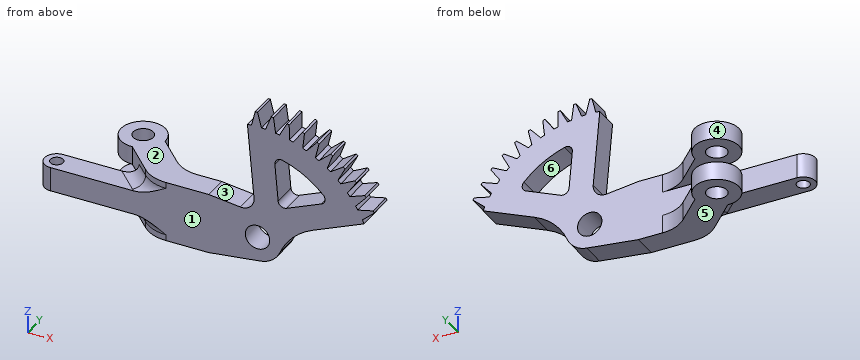
from build123d import *

# Parameters (mm, degrees)
SKETCH1_R           = 1.6500000000000001
BOSS_EXTRUDE1_DEPTH = 5
CUT_EXTRUDE1_DEPTH  = 22.617643257302586
SKETCH4_R           = 2.000000000000003
BOSS_EXTRUDE2_DEPTH = 4
SKETCH5_R           = 1.0500000000000005
BOSS_EXTRUDE3_DEPTH = 2
CUT_EXTRUDE2_REACH  = 52.658
CIRPATTERN1_COUNT   = 11
CIRPATTERN1_ANGLE   = 70.00000000000016
CUT_EXTRUDE3_DEPTH  = 4
FILLET1_R           = 6
FILLET2_R           = 2
CUT_EXTRUDE4_REACH  = 51.172


with BuildPart() as part:
    # Sketch1 → Boss-Extrude1 (new, symmetric)
    with BuildSketch(Plane.XY):
        with BuildLine():
            Line((6.464466094067297, -10), (16, -10))
            Line((16, -10), (16, -5.999999999999998))
            Line((16, -5.999999999999998), (9.535533905932775, -5.999999999999998))
            Line((9.535533905932775, -5.999999999999998), (3.6482589098755183, -0.11272500394276944))
            ThreePointArc((3.6482589098755183, -0.11272500394276944), (-2.580939751330903, 2.5809397513308943), (0.11272500394278592, -3.6482589098755174))
            Line((0.11272500394278592, -3.6482589098755174), (6.464466094067297, -10))
        make_face()
        Circle(SKETCH1_R, mode=Mode.SUBTRACT)
    extrude(amount=BOSS_EXTRUDE1_DEPTH, both=True)

    # Sketch3 → Cut-Extrude1 (cut, through all)
    with BuildSketch(Plane.XZ.offset(10)):
        Polygon((6.464466094067297, 2.000000000000001), (-3.6500000000000012, 1.9999999999999996), (-3.650000000000001, -2.0000000000000004), (6.464466094067298, -1.9999999999999991), align=None)
    extrude(amount=-CUT_EXTRUDE1_DEPTH, mode=Mode.SUBTRACT)

    # Sketch4 → Boss-Extrude2 (add)
    with BuildSketch(Plane.XZ.offset(10)):
        with BuildLine():
            Line((16, 5), (16, -5))
            Line((16, -5), (21.19546555409763, -4.369618467658506))
            Line((21.19546555409763, -4.369618467658506), (24.481798594453377, -3.970877751125406))
            ThreePointArc((24.481798594453377, -3.970877751125406), (26.41654324887739, -3.187525486377344), (27.693251449070946, -1.5361945625263))
            ThreePointArc((27.693251449070946, -1.5361945625263), (29.829731429750588, 1.668713133124987), (33.01906878685553, 3.8283675656823353))
            Line((33.01906878685553, 3.8283675656823353), (43.79085434922743, 8.400719262519475))
            ThreePointArc((43.79085434922743, 8.400719262519475), (35.07331861056618, 18.429096965095408), (22.126151530925494, 21.418186008972544))
            Line((22.126151530925494, 21.418186008972544), (23.428754247507808, 6.529368828716514))
            ThreePointArc((23.428754247507808, 6.529368828716514), (22.82671005925236, 4.917371632507108), (21.19546555409763, 4.369618467658506))
            Line((21.19546555409763, 4.369618467658506), (16, 5))
        make_face()
        with Locations(Location((24, 0, 0), (0, 0, 270))):
            Circle(SKETCH4_R, mode=Mode.SUBTRACT)
    extrude(amount=-BOSS_EXTRUDE2_DEPTH)

    # Sketch5 → Boss-Extrude3 (add, symmetric)
    with BuildSketch(Plane.XY):
        with BuildLine():
            Line((6.464466094067297, -10), (-10, -10.000000000000002))
            ThreePointArc((-10, -10.000000000000002), (-11.999999999999998, -8), (-9.999999999999998, -6.000000000000002))
            Line((-9.999999999999998, -6.000000000000002), (9.535533905932775, -5.999999999999998))
            Line((9.535533905932775, -5.999999999999998), (16, -5.999999999999998))
            Line((16, -5.999999999999998), (16, -10))
            Line((16, -10), (6.464466094067297, -10))
        make_face()
        with Locations((-9.999999999999998, -8.000000000000002)):
            Circle(SKETCH5_R, mode=Mode.SUBTRACT)
    extrude(amount=BOSS_EXTRUDE3_DEPTH, both=True)

    # Sketch6 → Cut-Extrude2 (cut, up to next)
    with BuildSketch(Plane.XZ.offset(10), mode=Mode.PRIVATE) as cut_extrude2_sk1:
        with BuildLine():
            Line((41.21984795369632, 8.029746973073365), (43.15664027004987, 9.760795744400328))
            ThreePointArc((43.15664027004987, 9.760795744400328), (43.324071995432064, 9.424979655965245), (43.48561742128794, 9.086292627425122))
            ThreePointArc((43.48561742128794, 9.086292627425122), (43.64122733931588, 8.744837826129787), (43.79085434922743, 8.40071926251947))
            ThreePointArc((43.79085434922743, 8.40071926251947), (43.93445287318589, 8.054041758442194), (44.071979169689804, 7.704910915224042))
            Line((44.071979169689804, 7.704910915224042), (41.48959221559633, 7.42389144129628))
            ThreePointArc((41.48959221559633, 7.42389144129628), (41.357363695209386, 7.72799621844028), (41.21984795369632, 8.029746973073365))
        make_face()
    cut_extrude2_tool1 = extrude(cut_extrude2_sk1.sketch, amount=-CUT_EXTRUDE2_REACH, mode=Mode.PRIVATE) & part.part
    cut_extrude2 = cut_extrude2_tool1.solids().sort_by_distance((42.701484, -10, 8.326437))[0]
    add(cut_extrude2, mode=Mode.SUBTRACT)

    # CirPattern1: Cut-Extrude2; each copy of Cut-Extrude2 runs up to whatever stops it at its own place
    cirpattern1_before = part.part  # the part as the pattern finds it: every copy runs up to it
    cirpattern1_cut_extrude2_long = extrude(cut_extrude2_sk1.sketch, amount=-CUT_EXTRUDE2_REACH, mode=Mode.PRIVATE)
    cirpattern1_cut_extrude2_tool1 = cirpattern1_cut_extrude2_long.rotate(Axis((24.000000000000014, 0, -2.52e-15), (0, -1, 0)), 1 * CIRPATTERN1_ANGLE / (CIRPATTERN1_COUNT - 1)) & cirpattern1_before
    add(cirpattern1_cut_extrude2_tool1.solids().sort_by_distance((41.547349, -10, 10.543511))[0], mode=Mode.SUBTRACT)
    cirpattern1_cut_extrude2_tool2 = cirpattern1_cut_extrude2_long.rotate(Axis((24.000000000000014, 0, -2.52e-15), (0, -1, 0)), 2 * CIRPATTERN1_ANGLE / (CIRPATTERN1_COUNT - 1)) & cirpattern1_before
    add(cirpattern1_cut_extrude2_tool2.solids().sort_by_distance((40.131623, -10, 12.603405))[0], mode=Mode.SUBTRACT)
    cirpattern1_cut_extrude2_tool3 = cirpattern1_cut_extrude2_long.rotate(Axis((24.000000000000014, 0, -2.52e-15), (0, -1, 0)), 3 * CIRPATTERN1_ANGLE / (CIRPATTERN1_COUNT - 1)) & cirpattern1_before
    add(cirpattern1_cut_extrude2_tool3.solids().sort_by_distance((38.475411, -10, 14.475411))[0], mode=Mode.SUBTRACT)
    cirpattern1_cut_extrude2_tool4 = cirpattern1_cut_extrude2_long.rotate(Axis((24.000000000000014, 0, -2.52e-15), (0, -1, 0)), 4 * CIRPATTERN1_ANGLE / (CIRPATTERN1_COUNT - 1)) & cirpattern1_before
    add(cirpattern1_cut_extrude2_tool4.solids().sort_by_distance((36.603405, -10, 16.131622))[0], mode=Mode.SUBTRACT)
    cirpattern1_cut_extrude2_tool5 = cirpattern1_cut_extrude2_long.rotate(Axis((24.000000000000014, 0, -2.52e-15), (0, -1, 0)), 5 * CIRPATTERN1_ANGLE / (CIRPATTERN1_COUNT - 1)) & cirpattern1_before
    add(cirpattern1_cut_extrude2_tool5.solids().sort_by_distance((34.543511, -10, 17.547348))[0], mode=Mode.SUBTRACT)
    cirpattern1_cut_extrude2_tool6 = cirpattern1_cut_extrude2_long.rotate(Axis((24.000000000000014, 0, -2.52e-15), (0, -1, 0)), 6 * CIRPATTERN1_ANGLE / (CIRPATTERN1_COUNT - 1)) & cirpattern1_before
    add(cirpattern1_cut_extrude2_tool6.solids().sort_by_distance((32.326437, -10, 18.701484))[0], mode=Mode.SUBTRACT)
    cirpattern1_cut_extrude2_tool7 = cirpattern1_cut_extrude2_long.rotate(Axis((24.000000000000014, 0, -2.52e-15), (0, -1, 0)), 7 * CIRPATTERN1_ANGLE / (CIRPATTERN1_COUNT - 1)) & cirpattern1_before
    add(cirpattern1_cut_extrude2_tool7.solids().sort_by_distance((29.985236, -10, 19.576823))[0], mode=Mode.SUBTRACT)
    cirpattern1_cut_extrude2_tool8 = cirpattern1_cut_extrude2_long.rotate(Axis((24.000000000000014, 0, -2.52e-15), (0, -1, 0)), 8 * CIRPATTERN1_ANGLE / (CIRPATTERN1_COUNT - 1)) & cirpattern1_before
    add(cirpattern1_cut_extrude2_tool8.solids().sort_by_distance((27.554808, -10, 20.160317))[0], mode=Mode.SUBTRACT)
    cirpattern1_cut_extrude2_tool9 = cirpattern1_cut_extrude2_long.rotate(Axis((24.000000000000014, 0, -2.52e-15), (0, -1, 0)), 9 * CIRPATTERN1_ANGLE / (CIRPATTERN1_COUNT - 1)) & cirpattern1_before
    add(cirpattern1_cut_extrude2_tool9.solids().sort_by_distance((25.071386, -10, 20.443268))[0], mode=Mode.SUBTRACT)
    cirpattern1_cut_extrude2_tool10 = cirpattern1_cut_extrude2_long.rotate(Axis((24.000000000000014, 0, -2.52e-15), (0, -1, 0)), 10 * CIRPATTERN1_ANGLE / (CIRPATTERN1_COUNT - 1)) & cirpattern1_before
    add(cirpattern1_cut_extrude2_tool10.solids().sort_by_distance((22.571993, -10, 20.421456))[0], mode=Mode.SUBTRACT)

    # Sketch7 → Cut-Extrude3 (cut)
    with BuildSketch(Plane(origin=(0, -5.999999999999998, 0), x_dir=(1, 0, 0), z_dir=(0, 1, 0))):
        Polygon((9.535533905932775, -2.0000000000000013), (6.464466094067297, -2.000000000000001), (6.464466094067298, 1.9999999999999991), (9.535533905932775, 1.9999999999999991), align=None)
    extrude(amount=CUT_EXTRUDE3_DEPTH, mode=Mode.SUBTRACT)

    # Fillet1
    fillet1_edges = [part.edges().sort_by_distance(p)[0] for p in [
        (6.464466094067297, -10, 3.5),
        (9.535533905932775, -5.999999999999998, 3.5),
        (6.464466094067297, -10, -3.4999999999999996),
        (9.535533905932775, -5.999999999999998, -3.5),
    ]]
    fillet(fillet1_edges, radius=FILLET1_R)

    # Fillet2
    # the kernel refuses this fillet: 2 mm, written as the material it adds along each edge
    with BuildSketch(Plane(origin=(-1.0710678118654662, -2.4644660940672707, -2), x_dir=(1.2e-16, -1e-17, -1), z_dir=(0.7071067811865491, -0.707106781186546, 0))) as fillet2_piece_1_section:
        with BuildLine():
            CenterArc((FILLET2_R, -FILLET2_R), FILLET2_R, 90, 90)
            Line((-1.6e-16, -FILLET2_R), (0, 0))
            Line((0, 0), (FILLET2_R, 0))
        make_face()
    fillet2_piece_1 = extrude(amount=8.171572875253831, mode=Mode.PRIVATE)
    fillet2_piece_1 = split(fillet2_piece_1, bisect_by=Plane(origin=(3.0707262538263027, -5.999999999999999, -2.423870706471317), z_dir=(1.8e-16, -1, 0)), keep=Keep.TOP, mode=Mode.PRIVATE)
    add(fillet2_piece_1)
    with BuildSketch(Plane(origin=(8.94974746830586, -3.999999999999999, -2), x_dir=(-0.7071067811865458, -0.7071067811865492, 0), z_dir=(-0.7071067811865492, 0.7071067811865458, 0))) as fillet2_piece_2_section:
        with BuildLine():
            CenterArc((6 + FILLET2_R, -FILLET2_R), FILLET2_R, 90, 90)
            Line((6 + FILLET2_R, 0), (6, 0))
            Line((6, 0), (6.000000000000001, -FILLET2_R))
        make_face()
    fillet2_piece_2 = revolve(axis=Axis((8.94974746830586, -3.999999999999999, -2), (0, 0, 1)), revolution_arc=92.75127695444853, mode=Mode.PRIVATE)
    fillet2_piece_2 = split(fillet2_piece_2, bisect_by=Plane(origin=(6.6265116676217675, -10, -2.6906159544544805), z_dir=(0, 1, 0)), keep=Keep.TOP, mode=Mode.PRIVATE)
    add(fillet2_piece_2)
    with BuildSketch(Plane(origin=(8.94974746830586, -3.999999999999999, 2), x_dir=(-0.7071067811865458, -0.7071067811865492, 0), z_dir=(-0.7071067811865492, 0.7071067811865458, 0))) as fillet2_piece_3_section:
        with BuildLine():
            CenterArc((6 + FILLET2_R, FILLET2_R), FILLET2_R, 180, 90)
            Line((6 + FILLET2_R, 0), (6, 0))
            Line((6, 0), (6.000000000000001, FILLET2_R))
        make_face()
    fillet2_piece_3 = revolve(axis=Axis((8.94974746830586, -3.999999999999999, 2), (0, 0, 1)), revolution_arc=92.75127695444853, mode=Mode.PRIVATE)
    fillet2_piece_3 = split(fillet2_piece_3, bisect_by=Plane(origin=(6.626511667621772, -10, 2.6906159544544797), z_dir=(0, 1, 0)), keep=Keep.TOP, mode=Mode.PRIVATE)
    add(fillet2_piece_3)
    with BuildSketch(Plane(origin=(4.707106781186583, -8.242640687119295, 2.0000000000000004), x_dir=(1.6e-16, 2.9e-16, 1), z_dir=(-0.7071067811865491, 0.707106781186546, 0))) as fillet2_piece_4_section:
        with BuildLine():
            CenterArc((FILLET2_R, -FILLET2_R), FILLET2_R, 89.99999999999999, 90.00000000000001)
            Line((-1.07e-15, -FILLET2_R), (0, 0))
            Line((0, 0), (FILLET2_R, 0))
        make_face()
    fillet2_piece_4 = extrude(amount=8.171572875253833, mode=Mode.PRIVATE)
    fillet2_piece_4 = split(fillet2_piece_4, bisect_by=Plane(origin=(3.0707262538259545, -5.999999999999999, 2.4238707064714085), z_dir=(1.8e-16, -1, 0)), keep=Keep.TOP, mode=Mode.PRIVATE)
    add(fillet2_piece_4)

    # Sketch8 → Cut-Extrude4 (cut, up to next)
    with BuildSketch(Plane(origin=(0, -5.999999999999998, 0), x_dir=(1, 0, 0), z_dir=(0, 1, 0)), mode=Mode.PRIVATE) as cut_extrude4_sk1:
        with BuildLine():
            ThreePointArc((28.115640284464295, -14.42433724816827), (31.725571123650823, -12.857509510531676), (34.803757775643525, -10.405710832289252))
            ThreePointArc((34.803757775643525, -10.405710832289252), (35.06330097352167, -9.511986093117567), (34.47423838575658, -8.791491923350865))
            Line((34.47423838575658, -8.791491923350865), (28.771906676032494, -6.370995718899502))
            ThreePointArc((28.771906676032494, -6.370995718899502), (27.866137472633152, -6.434333271649826), (27.38498084945146, -7.2043448296042945))
            Line((27.38498084945146, -7.2043448296042945), (26.845069567408263, -13.375559022209401))
            ThreePointArc((26.845069567408263, -13.375559022209401), (27.20468002661588, -14.23392193997834), (28.115640284464295, -14.42433724816827))
        make_face()
    cut_extrude4_tool1 = extrude(cut_extrude4_sk1.sketch, amount=-CUT_EXTRUDE4_REACH, mode=Mode.PRIVATE) & part.part
    add(cut_extrude4_tool1.solids().sort_by_distance((30.212176, -6, 10.338796))[0], mode=Mode.SUBTRACT)


solid = part.part
Input: part model. Units: mm. Frame: model coordinates. Face numbers are marked on the shaded views. A direction names the side the tool comes from. Give positions to 0.01 mm unless a question says otherwise; leave off trailing zeros. Loops run counter-clockwise (first coordinate to the right, second up) from the corner with the lowest first, then second, coordinate; pieces in that order, holes last. Notation, with made-up numbers: (-2.75, -7.5) - (16.25, -7.5) arc R15 cw to (16.25, -3.5) - close; hole circle Ø6 at (67.25, -36). An arc over 180 degrees is marked (long way). Use CSV: the item, a comma, the result in double quotes. Start each with the question number.
Item 1: Section B-B on y = 2.25. Return loops of the section in (x, z), then the cut area to 3 significant figures.
Item 2: Mould query, pull axis X, two halves, no side actions, for the marked faces 4, 5 and 6. Classes: pulls with the +X half, pulls with the -X half, needs draft (parallel to the pull), parting line crosses it, or undercut.
Item 3: Reachability of the marked faces 1, 2 and 3 from +Z, -Z, +X, -X, +Y, -Y: full face, straight path, thin tool, end or side. Return the list, or none.
Item 4: Section C-C on y = -5. Return loops of the section in (x, z), then the cut area to 3 significant figures.
Item 5: Contact query for flat-ended pins moving along their axis: P1, Ø3, axis at x = 0, y = 0, coming from the -Z side; P2, Ø4.5, axis at x = -7, y = -7.5, coming from the +Z side; P3, Ø7.5, axis at x = 1, y = 0, coming from the +Z side; P4, Ø2, axis at x = -2.5, y = -7.5, coming from the -Z side. Output: stop coordinate, or through.
Item 6: Line query: line 1 (Y direction, x = 0, z = -3.8); line 2 (X direction, y = -7.5, z = 0). Output: solid intervals per line, ascending.
Item 7: Section A-A on z = 0. Return loops of the section in (x, y), then the cut area to 3 significant figures.
Ans:
1,outline,"(-2.87, -5) - (2.87, -5) - (2.87, -2) - (-2.87, -2) - close; (-2.87, 2) - (2.87, 2) - (2.87, 5) - (-2.87, 5) - close"
1,area,"34.5 mm2"
2,face 4,"parting line crosses it"
2,face 5,"needs draft"
2,face 6,"undercut"
3,face 1,"+Z, -Z, +X, -X, -Y"
3,face 2,"+Z, -X, +Y, -Y"
3,face 3,"+Z, +Y, -Y"
4,outline,"(1.46, -5) - (8.7, -5) - (8.7, -2) - (1.46, -2) - close; (1.46, 2) - (8.7, 2) - (8.7, 5) - (1.46, 5) - close"
4,area,"43.4 mm2"
5,P1,"passes through"
5,P2,"stops at z = 2"
5,P3,"stops at z = 5"
5,P4,"stops at z = -2"
6,line 1,"y = -3.65 to -1.65, 1.65 to 3.65"
6,line 2,"x = -11.94 to -10.92, -9.08 to 22, 26 to 28.49"
7,outline,"(-10, -10) - (22, -10) - (22, -6) - (-10, -6) arc R2 ccw to start; (26, -10) - (28.49, -10) - (28.49, -6) - (26, -6) - close; hole circle Ø2.1 at (-10, -8)"
7,area,"141 mm2"
